For this review, take the finished solid that the model builds, in its own axes (mm). A direction names the side the tool comes from. Give positions to 0.01 mm unless a question says otherwise; leave off trailing zeros. Write each loop counter-clockwise with the first axis right and the second up, starting at its lowest first coordinate (ties: lowest second). Pieces come first, ordered by that corner, then holes.
Autodesk Inventor part; units mm, degrees
ref_plane "YZ Plane" through (0, 0, 0) normal (1, 0, 0) x (0, 1, 0)
ref_plane "XZ Plane" through (0, 0, 0) normal (0, 1, 0) x (-1, 0, 0)
ref_plane "XY Plane" through (0, 0, 0) normal (0, 0, 1) x (1, 0, 0)
sketch "Sketch1" plane through (0, 0, 0) normal (0, 0, 1) x (1, 0, 0)
  line L0 (0, 0) -> (102.5, 0)
  line L1 (0, 0) -> (0, 16)
  line L2 (0, 4.2898) -> (79, 4.2898)
  line L3 (79, 4.2898) -> (79, 6)
  line L4 (79, 6) -> (92.5, 6)
  line L5 (92.5, 6) -> (92.5, 0)
  line L6 (0, 16) -> (102.5, 16)
  line L7 (102.5, 16) -> (102.5, 0)
  circle A0 centre (97.5, 11) radius 1.5875
  dimension "d0" = 13.5
  dimension "d1" = 12
  dimension "d2" = 8.5796
  dimension "d3" = 185
  dimension "d4" = 10
  dimension "d5" = 10
  dimension "d6" = 3.175
  dimension "d7" = 5
  dimension "d8" = 5
extrude "Extrusion1" add sketch "Sketch1" along normal blind 6.35 contours L5 L4 L3 L2 L1 L6 L7 L0
sketch "Sketch2" plane through (0, 0, 6.35) normal (0, 0, 1) x (1, 0, 0)
  line L0 (79, 4.2898) -> (79, 6)
  line L1 (79, 6) -> (92.5, 6)
  line L2 (92.5, 6) -> (92.5, 0)
  arc A0 (82.175, 6) -> (79, 6) centre (80.5875, 6) ccw
  arc A1 (92.5, 6) -> (89.325, 6) centre (90.9125, 6) ccw
  point P0 (0, 0)
  dimension "d12" = 1.5875
extrude "Extrusion2" cut sketch "Sketch2" against normal up to next
fillet "Fillet1" radius 2 1 edges at (102.5, 16, 3.175)
mirror "Mirror1" about plane through (92.5, 0, 0) normal (0, -1, 0) of "Extrusion1", "Fillet1", "Extrusion2"
mirror "Mirror2" about plane through (0, -16, 0) normal (-1, 0, 0) of "Extrusion1", "Fillet1", "Mirror1", "Extrusion2"
properties part number "Arrow_Arm_Template"
(1) We need section B-B (y = -1). Write out the cut boundary in (x, z), and give its area (3 significant figures).
(2) Tool access review of faces 1 (the flat face through (0, -16, 3)), 2 (the flat face through (-86, -6, 3)): name each direction out of +Z, -Z, +X, -X, +Y, -Y from which nothing blocks a thin tool from reaching the whole face with its end or side.
(3) We need section A-A (x = 52). Write out the cut boundary in (y, z), and give its area (3 significant figures).
(4) The part is to be moulded in two halves that separate along Y. For faces 3 (the cylindrical face through (-80.553, 7.587, 3.219)), 4 (the flat face through (-92.5, 0, 3)), 5 (the flat face through (-1, 16, 3)), 6 (the flat face through (1, -7, 6.35)), say which applies: +Y half, -Y half, draft (parallel to the pull), parting line (faces both ways), or undercut.
(5) For L1, parallel to X at y = 5, z = 3.5; L2, parallel to Y at x = -97.5, z = 4.25; L3, parallel to X at y = -11, z = 3.75, list the stretches that pass through material, from the lowest coordinate up.
The answers:
1. outline: (-102.5, 0) - (-92.5, 0) - (-92.5, 6.35) - (-102.5, 6.35) - close; (92.5, 0) - (102.5, 0) - (102.5, 6.35) - (92.5, 6.35) - close
1. area: 127 mm2
2. face 1: +Z, -Z, +X, -X, -Y
2. face 2: +Z, -Z
3. outline: (-16, 0) - (-4.29, 0) - (-4.29, 6.35) - (-16, 6.35) - close; (4.29, 0) - (16, 0) - (16, 6.35) - (4.29, 6.35) - close
3. area: 149 mm2
4. face 3: undercut
4. face 4: undercut
4. face 5: +Y half
4. face 6: draft
5. L1: x = -102.5 to -92.5, -79 to 79, 92.5 to 102.5
5. L2: y = -16 to -12.59, -9.41 to 9.41, 12.59 to 16
5. L3: x = -102.5 to -99.09, -95.91 to 95.91, 99.09 to 102.5
